```python
from build123d import *

# Parameters (mm, degrees)
ESQUISSE1_R                  = 5.75
ESQUISSE1_R_2                = 1.6
BOSS_EXTRU_1_DEPTH           = 5.25
ESQUISSE2_R                  = 3
ENL_V_MAT_EXTRU_1_DEPTH      = 3
ENL_V_START                  = -3
ESQUISSE3_R                  = 5.75
ESQUISSE3_R_2                = 4.5
ENL_V_MAT_EXTRU_2_DEPTH      = 3
BOSS_EXTRU_2_DEPTH           = 2.25
R_P_TITION_CIRCULAIRE1_COUNT = 2
ESQUISSE5_R                  = 0.75
ENL_V_MAT_EXTRU_3_DEPTH      = 3
R_P_TITION_CIRCULAIRE2_COUNT = 2
BOSS_EXTRU_3_DEPTH           = 3
R_P_TITION_CIRCULAIRE3_COUNT = 28
ENL_V_START_2                = -1
ESQUISSE7_R                  = 3
ESQUISSE7_R_2                = 1.6
ENL_V_MAT_EXTRU_4_DEPTH      = 1
ESQUISSE8_R                  = 4.7
ESQUISSE8_R_2                = 3.4
ENL_V_MAT_EXTRU_5_DEPTH      = 1


with BuildPart() as part:
    # Esquisse1 → Boss.-Extru.1 (new body)
    with BuildSketch(Plane.XY):
        with Locations(Location((0, 0, 0), (0, 0, 180))):
            Circle(ESQUISSE1_R)
        with Locations(Location((0, 0, 0), (0, 0, 180))):
            Circle(ESQUISSE1_R_2, mode=Mode.SUBTRACT)
    extrude(amount=BOSS_EXTRU_1_DEPTH)

    # Esquisse2 → Enlèv. mat.-Extru.1 (cut)
    with BuildSketch(Plane.XY.offset(5.25)):
        Circle(ESQUISSE2_R)
    extrude(amount=-ENL_V_MAT_EXTRU_1_DEPTH, mode=Mode.SUBTRACT)

    # Esquisse3 → Enlèv. mat.-Extru.2 (cut)
    with BuildSketch(Plane.XY.offset(5.25).offset(ENL_V_START)):
        with Locations(Location((0, 0, 0), (0, 0, 180))):
            Circle(ESQUISSE3_R)
        Circle(ESQUISSE3_R_2, mode=Mode.SUBTRACT)
    extrude(amount=ENL_V_MAT_EXTRU_2_DEPTH, mode=Mode.SUBTRACT)

    # Esquisse4 → Boss.-Extru.2 (add)
    with BuildSketch(Plane(origin=(0, 0, 0), x_dir=(-1, 0, 0), z_dir=(0, 0, -1))):
        with BuildLine():
            Line((-4.3, 3.817394399), (-2.475852955, 16.846629695))
            ThreePointArc((-2.475852955, 16.846629695), (0, 19), (2.475852955, 16.846629695))
            Line((2.475852955, 16.846629695), (4.3, 3.817394399))
            ThreePointArc((4.3, 3.817394399), (0, 5.75), (-4.3, 3.817394399))
        make_face()
    boss_extru_2 = extrude(amount=-BOSS_EXTRU_2_DEPTH)

    # Répétition circulaire1: Boss.-Extru.2 ×2 about axis
    r_p_tition_circulaire1_axis = Axis((0, 0, 0), (0, 0, 1))
    for i in range(1, R_P_TITION_CIRCULAIRE1_COUNT):
        add(boss_extru_2.rotate(r_p_tition_circulaire1_axis, i * 360 / R_P_TITION_CIRCULAIRE1_COUNT))

    # Esquisse5 → Enlèv. mat.-Extru.3 (cut)
    with BuildSketch(Plane(origin=(0, 0, 0), x_dir=(-1, 0, 0), z_dir=(0, 0, -1))):
        with Locations((0, 7.25)):
            Circle(ESQUISSE5_R)
        with Locations((0, 10.25)):
            Circle(ESQUISSE5_R)
        with Locations((0, 13.25)):
            Circle(ESQUISSE5_R)
        with Locations((0, 16.25)):
            Circle(ESQUISSE5_R)
    enl_v_mat_extru_3 = extrude(amount=-ENL_V_MAT_EXTRU_3_DEPTH, mode=Mode.SUBTRACT)

    # Répétition circulaire2: Enlèv. mat.-Extru.3 ×2 about axis
    r_p_tition_circulaire2_axis = Axis((0, 0, 0), (0, 0, 1))
    for i in range(1, R_P_TITION_CIRCULAIRE2_COUNT):
        add(enl_v_mat_extru_3.rotate(r_p_tition_circulaire2_axis, i * 360 / R_P_TITION_CIRCULAIRE2_COUNT), mode=Mode.SUBTRACT)

    # Esquisse6 → Boss.-Extru.3 (add)
    with BuildSketch(Plane.XY.offset(5.25)):
        Polygon((-0.3, 3), (0, 2.7), (0.3, 3), align=None)
    boss_extru_3 = extrude(amount=-BOSS_EXTRU_3_DEPTH)

    # Répétition circulaire3: Boss.-Extru.3 ×28 about axis
    r_p_tition_circulaire3_axis = Axis((0, 0, 0), (0, 0, 1))
    for i in range(1, R_P_TITION_CIRCULAIRE3_COUNT):
        add(boss_extru_3.rotate(r_p_tition_circulaire3_axis, i * 360 / R_P_TITION_CIRCULAIRE3_COUNT))

    # Esquisse7 → Enlèv. mat.-Extru.4 (cut)
    with BuildSketch(Plane(origin=(0, 0, 0), x_dir=(-1, 0, 0), z_dir=(0, 0, -1)).offset(ENL_V_START_2)):
        Circle(ESQUISSE7_R)
        Circle(ESQUISSE7_R_2, mode=Mode.SUBTRACT)
    extrude(amount=ENL_V_MAT_EXTRU_4_DEPTH, mode=Mode.SUBTRACT)

    # Esquisse8 → Enlèv. mat.-Extru.5 (cut)
    with BuildSketch(Plane(origin=(0, 0, 0), x_dir=(-1, 0, 0), z_dir=(0, 0, -1))):
        Circle(ESQUISSE8_R)
        Circle(ESQUISSE8_R_2, mode=Mode.SUBTRACT)
    extrude(amount=-ENL_V_MAT_EXTRU_5_DEPTH, mode=Mode.SUBTRACT)


solid = part.part
```
Here's how the part is built. I have some questions about the finished solid (model axes, mm). A direction names the side the tool comes from. Give positions to 0.01 mm unless a question says otherwise; leave off trailing zeros. Order: outer loops, then holes, each group sorted by start corner. A loop starts at its lowest first (then second) coordinate and runs counter-clockwise, first axis right, second up. Notation, with made-up numbers: (73.25, 89.5) - (112.25, 89.5) arc R15 ccw to (112.25, 110.5) - close; hole circle Ø5 at (87.5, 46). An arc over 180 degrees is marked (long way). Answer as a JSON object with one key per item and string values. Group by question number.
Item 1: If we mould it in two halves opening along X, with no side actions, what happens to faces 1 (the flat face through (-3.375, 10.423, 1.109)), 2 (the cylindrical face through (0, -19, 1)), 3 (the cylindrical face through (0.74, -3.32, 0.49)), 4 (the flat face through (1.3, -1.3, 2.25))? For each: pulls with the +X half, pulls with the -X half, needs draft (parallel to the pull), parting line crosses it, or undercut.
Item 2: If we section it at B-B on y = 7.25: Please give me the cut outline in (x, z), and give its area (3 significant figures).
Item 3: Which directions (+Z, -Z, +X, -X, +Y, -Y) give clear straight access to the entire face, cutting with the end or side of a thin tool? Please do faces 5 (the flat face through (-1.2, -4.5, 2.25)), 6 (the cylindrical face through (1.02, -4.59, 0.49)), 7 (the cylindrical face through (0, -11, 1)).
Item 4: For P1, Ø5, axis at x = 0, y = 0, coming from the -Z side; P2, Ø3, axis at x = -2, y = 8.5, coming from the +Z side; P3, Ø0.9, axis at x = 0, y = 10.25, coming from the -Z side; P4, Ø3, axis at y = -6, z = 1, coming from the -X side, each with a flat end and sliding along its axis, tell me the tip position at first contact or that it passes through.
Item 5: If we section it at C-C on y = -10.25: Please give me the cut outline in (x, z), and give its area (3 significant figures).
Item 6: If we section it at A-A on z = 0.5: Give the number of separate pieces and of enclosed holes in the cut face, and give its area (3 significant figures).
Item 7: If we section it at D-D on y = 11.5: Please give me the cut outline in (x, z).
Item 8: Please list where these lines run through material, in increasing order: probe 1 along X at (y, z) = (-7.25, 1.5); probe 2 along Z at (x, y) = (-2.75, -5); probe 3 along X at (y, z) = (-10.25, 0.75).
Result set:
{
 "1": {"face 1": "pulls with the -X half", "face 2": "parting line crosses it", "face 3": "undercut", "face 4": "undercut"},
 "2": {"outline": "(-3.82, 0) - (-0.75, 0) - (-0.75, 2.25) - (-3.82, 2.25) - close; (0.75, 0) - (3.82, 0) - (3.82, 2.25) - (0.75, 2.25) - close", "area": "13.8 mm²"},
 "3": {"face 5": "+Z", "face 6": "-Z", "face 7": "+Z, -Z"},
 "4": {"P1": "z = 1", "P2": "z = 2.25", "P3": "through", "P4": "x = -4.2"},
 "5": {"outline": "(-3.4, 0) - (-0.75, 0) - (-0.75, 2.25) - (-3.4, 2.25) - close; (0.75, 0) - (3.4, 0) - (3.4, 2.25) - (0.75, 2.25) - close", "area": "11.9 mm²"},
 "6": {"separate pieces": "2", "enclosed holes": "10", "area": "198 mm²"},
 "7": {"outline": "(-3.22, 0) - (3.22, 0) - (3.22, 2.25) - (-3.22, 2.25) - close"},
 "8": {"probe 1": "-3.82 to -0.75, 0.75 to 3.82", "probe 2": "0 to 2.25", "probe 3": "-3.4 to -0.75, 0.75 to 3.4"}
}
